from build123d import *

# Parameters (mm, degrees)
BOSS_EXTRUDE1_DEPTH                   = 3.175
F_16_0_177_DIAMETER_HOLE1_D           = 4.4958
F_16_0_177_DIAMETER_HOLE1_DEPTH       = 3.175
F_16_0_177_DIAMETER_HOLE1_CSINK_D     = 5.7658
F_16_0_177_DIAMETER_HOLE1_CSINK_ANGLE = 100
F_16_0_177_DIAMETER_HOLE1_TIP         = 1.350674586


with BuildPart() as part:
    # Sketch1 → Boss-Extrude1 (new body)
    with BuildSketch(Plane(origin=(0, 0, 0), x_dir=(1, 0, 0), z_dir=(0, 1, 0))):
        Polygon((-137.16, -50.8), (137.16, -50.8), (137.16, -22.86), (165.1, -22.86), (165.1, 101.6), (-165.1, 101.6), (-165.1, -22.86), (-137.16, -22.86), align=None)
    extrude(amount=BOSS_EXTRUDE1_DEPTH)

    # #16 (0.177) Diameter Hole1
    with Locations(Plane(origin=(0, 3.175, 0), x_dir=(1, 0, 0), z_dir=(0, 1, 0))):
        with Locations((-47.752, 50.8), (-25.4, 50.8), (-25.4, 28.448), (-47.752, 28.448), (25.4, 28.448), (25.4, 50.8), (47.752, 50.8), (47.752, 28.448)):
            CounterSinkHole(F_16_0_177_DIAMETER_HOLE1_D / 2, F_16_0_177_DIAMETER_HOLE1_CSINK_D / 2, depth=F_16_0_177_DIAMETER_HOLE1_DEPTH, counter_sink_angle=F_16_0_177_DIAMETER_HOLE1_CSINK_ANGLE)
            with Locations((0, 0, -(F_16_0_177_DIAMETER_HOLE1_DEPTH + F_16_0_177_DIAMETER_HOLE1_TIP / 2))):  # 118° drill point
                Cone(0, F_16_0_177_DIAMETER_HOLE1_D / 2, F_16_0_177_DIAMETER_HOLE1_TIP, mode=Mode.SUBTRACT)


solid = part.part
Here's how the part is built. I have some questions about the finished solid (model axes, mm). Give positions to 0.01 mm unless a question says otherwise; leave off trailing zeros. Order: outer loops, then holes, each group sorted by start corner. A loop starts at its lowest first (then second) coordinate and runs counter-clockwise, first axis right, second up. Notation, with made-up numbers: M 7,68.5 L 17,68.5 A24 ccw 17,78.5 Z; hole C 68.25,19 d1. An arc over 180 degrees is marked long. Answer as a JSON object with one key per item and string values. Group by question number.
1) Suppose I cut it at A-A, the plane y = 1. Count the separate pieces of the cut face and the enclosed holes in it, plus the area to 3 significant figures.
2) We'd pull the mould along X, two halves only. Please class faces 1 (the flat face through (-2, 0, -26)), 2 (the conical face through (50, 3, -27)): pulls with the +X half, pulls with the -X half, needs draft (parallel to the pull), parting line crosses it, or undercut.
3) Please list where these lines run through material, in increasing order: L1, parallel to X at y = 1.05, z = -50.8; L2, parallel to Z at x = 46, y = 2; L3, parallel to Z at x = 151, y = 0.5. Write a range as [from, to].
4) I'm going to push a flat-ended pin straight in: pin 1 Ø3.5 at (x, z) = (-25.4, -50.8) entering from -Y. Where does the tip first touch, or does it pass through?
5) Suppose I cut it at B-B, the plane x = -143. Write out the boundary of the cut face in (y, z) (3 decimals).
Results found:
{
 "1": {"separate pieces": "1", "enclosed holes": "8", "area": "48,600 mm²"},
 "2": {"face 1": "needs draft", "face 2": "undercut"},
 "3": {"L1": "[-165.1, -50], [-45.5, -27.65], [-23.15, 23.15], [27.65, 45.5], [50, 165.1]", "L2": "[-101.6, -52.21], [-49.39, -29.86], [-27.04, 50.8]", "L3": "[-101.6, 22.86]"},
 "4": {"pin 1": "through"},
 "5": {"outline": "M 0,-101.6 L 3.175,-101.6 L 3.175,22.86 L 0,22.86 Z"}
}
